Geometry check sheet. Reference: drawing and pictorial views, mm from the part's lowest x, y, z. Coordinates: 2 decimals unless noted, no trailing zeros. Write each loop counter-clockwise with the first axis right and the second up, starting at its lowest first coordinate (ties: lowest second). Pieces come first, ordered by that corner, then holes. Notation, with made-up numbers: (75, -29.5) -> (87, -29.5) arc R20 cw to (87, 2.5) -> close; hole circle Ø3 at (24, 44). An arc over 180 degrees is marked (long way). Answer in a Markdown table with one row per item.
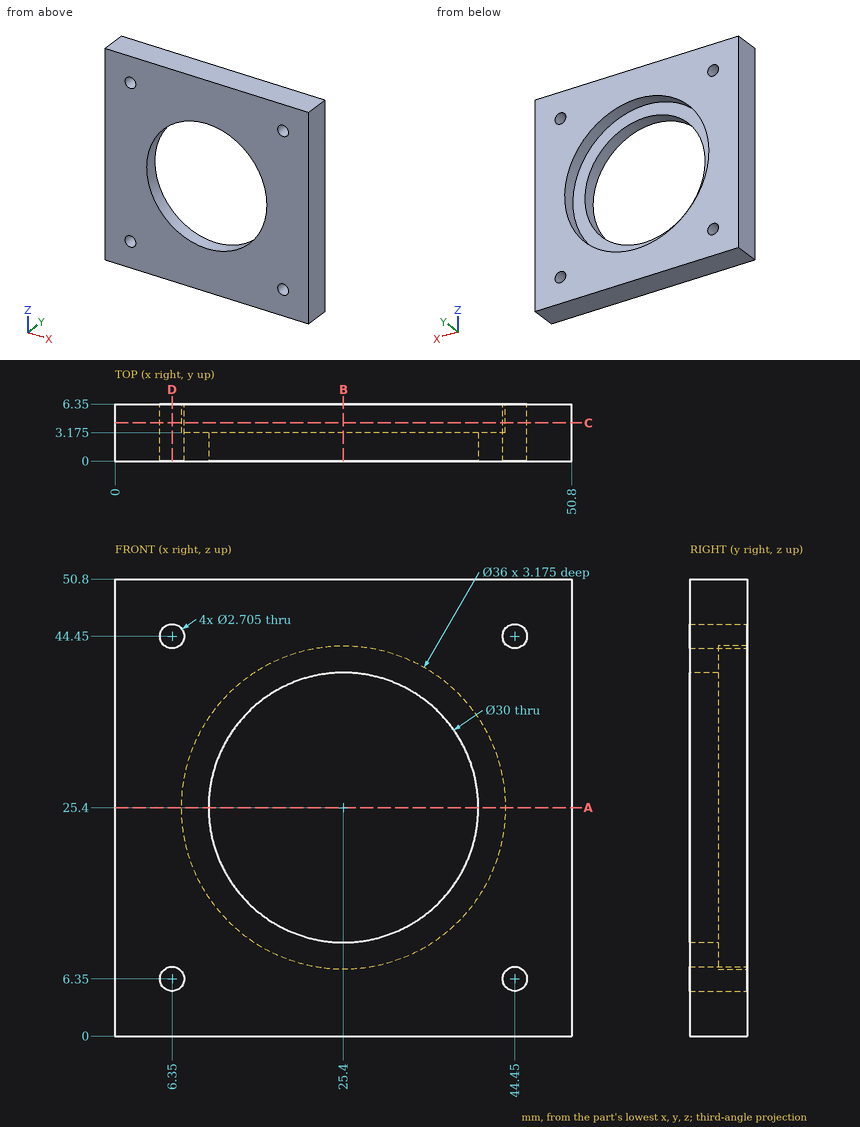
1. Section check C-C, the plane y = 4.25. State how many separate pieces and enclosed holes the cut face has, plus the area to 3 significant figures.
Geometry says:
| item | result |
|---|---|
| separate pieces | 1 |
| enclosed holes | 5 |
| area | 1,540 mm^2 |
2. Section check A-A, the plane z = 25.4. Record the boundary of the cut face in (x, y) (3 decimals).
Geometry says:
| item | result |
|---|---|
| outline | (0, 0) -> (10.4, 0) -> (10.4, 3.175) -> (7.4, 3.175) -> (7.4, 6.35) -> (0, 6.35) -> close; (40.4, 0) -> (50.8, 0) -> (50.8, 6.35) -> (43.4, 6.35) -> (43.4, 3.175) -> (40.4, 3.175) -> close |
3. Section check B-B, the plane x = 25.4. Record the boundary of the cut face in (y, z) (3 decimals), plus the area to 3 significant figures.
Geometry says:
| item | result |
|---|---|
| outline | (0, 0) -> (6.35, 0) -> (6.35, 7.4) -> (3.175, 7.4) -> (3.175, 10.4) -> (0, 10.4) -> close; (0, 40.4) -> (3.175, 40.4) -> (3.175, 43.4) -> (6.35, 43.4) -> (6.35, 50.8) -> (0, 50.8) -> close |
| area | 113 mm^2 |
4. Depth check by flat-ended pin: P1, Ø2.5, axis at x = 44.45, z = 6.35, coming from the -Y side; P2, Ø4.5, axis at x = 6.35, z = 44.45, coming from the -Y side. Enter the tip coordinate at first touch or a pass-through.
Geometry says:
| item | result |
|---|---|
| P1 | through |
| P2 | y = 0 |
5. Section check D-D, the plane x = 6.35. Record the boundary of the cut face in (y, z).
Geometry says:
| item | result |
|---|---|
| outline | (0, 0) -> (6.35, 0) -> (6.35, 5) -> (0, 5) -> close; (0, 7.7) -> (6.35, 7.7) -> (6.35, 43.1) -> (0, 43.1) -> close; (0, 45.8) -> (6.35, 45.8) -> (6.35, 50.8) -> (0, 50.8) -> close |
6. Thickness scan on line 1 (Z direction, x = 44.45, y = 5.25); line 2 (X direction, y = 1.25, z = 44). Record the ranges inside material, lowest first. Write a range as from..to.
Geometry says:
| item | result |
|---|---|
| line 1 | 0..5, 7.7..43.1, 45.8..50.8 |
| line 2 | 0..5.07, 7.63..43.17, 45.73..50.8 |
